```python
from build123d import *

# Parameters (mm, degrees)
SKETCH_2_R          = 4.5
CUT_EXTRUDE_1_DEPTH = 73.498275842


with BuildPart() as part:
    # 草图1 one side → 旋转4 (revolve)
    with BuildSketch(Plane(origin=(0, 0, 0), x_dir=(1, 0, 0), z_dir=(0, 1, 0)), mode=Mode.PRIVATE) as revolve_4_sk:
        with BuildLine():
            Line((0, 10), (-20.468871126, 10))
            ThreePointArc((-20.468871126, 10), (-23.116081379, 11.001287297), (-24.437982633, 13.503861062))
            Line((-24.437982633, 13.503861062), (-26, 26))
            Line((-26, 26), (-31, 26))
            Line((-31, 26), (-31, 10))
            Line((-31, 10), (-50, 10))
            Line((-50, 10), (-50, -2))
            Line((-50, -2), (-31, -2))
            Line((-31, -2), (-31, 0))
            Line((-31, 0), (0, 0))
            Line((0, 0), (0, 10))
        make_face()
    revolve(revolve_4_sk.sketch.rotate(Axis((0, 0, 0), (0, 0, -1)), 180), axis=Axis((0, 0, 0), (0, 0, -1)))

    # 草图2 → 切除-拉伸1 (cut, through all)
    with BuildSketch(Plane(origin=(0, 0, -10), x_dir=(-1, 0, 0), z_dir=(0, 0, -1))):
        with Locations((41, 0)):
            Circle(SKETCH_2_R)
        with Locations((0, -41)):
            Circle(SKETCH_2_R)
        with Locations((-41, 0)):
            Circle(SKETCH_2_R)
        with Locations((0, 41)):
            Circle(SKETCH_2_R)
    extrude(amount=-CUT_EXTRUDE_1_DEPTH, mode=Mode.SUBTRACT)


solid = part.part
```
Here's how the part is built. I have some questions about the finished solid (model axes, mm). A direction names the side the tool comes from. Coordinates: 2 decimals unless noted, no trailing zeros. Order: outer loops, then holes, each group sorted by start corner. A loop starts at its lowest first (then second) coordinate and runs counter-clockwise, first axis right, second up. Notation, with made-up numbers: (74, -31.75) - (88, -31.75) arc R22 ccw to (88, -4.75) - close; hole circle Ø11 at (18.5, -35). An arc over 180 degrees is marked (long way). One line per question, with ' | ' between items. Start each with the question number.
1. I'm going to push flat-ended pins straight in: pin 1 Ø1 at (x, z) = (16, -8.5) entering from +Y; pin 2 Ø1 at (x, z) = (24, -13) entering from +Y; pin 3 Ø6 at (x, y) = (17.5, 32.5) entering from -Z; pin 4 Ø7 at (x, y) = (41, 0) entering from -Z. Where does each tip first touch, or does it pass through?
2. If we section it at D-D (y = 43): Write out the boundary of the cut face in (x, z), and give its area (3 significant figures).
3. If we mould it in two halves opening along Z, with no side actions, what happens to faces 1 (the cylindrical face through (-4.036, -30.736, 0.986)), 2 (the flat face through (22, -23, 2)), 3 (the flat face through (16, 21, -26))? For each: released by +Z, released by -Z, zero draft, split by the parting line, or undercut.
4. Please list where these lines run through material, in increasing order: line 1 along Y through (x, z) = (0, 1.3); line 2 along Z through (x, y) = (-15.5, 12.5); line 3 along Z through (x, y) = (22.5, -39). Write a range as [from, to].
5. If we section it at A-A (x = 0): Write out the boundary of the cut face in (y, z), and give its area (3 significant figures).
6. Which directions (+Z, -Z, +X, -X, +Y, -Y) give clear straight access to the entire face, cutting with the end or side of a thin tool? Please do faces 4 (the flat face through (0, 0, 0)), 5 (the flat face through (0, 0, -10)), 6 (the cylindrical face through (36.708, 1.352, -4.084)).
7. If we section it at B-B (z = -2.5): Write out the boundary of the cut face in (x, y), and give its area (3 significant figures).
Model answer:
1) pin 1: stops at y = 47.54 | pin 2: stops at y = 20.22 | pin 3: stops at z = -10 | pin 4: passes through
2) outline: (-25.51, -10) - (-4.03, -10) - (-4.03, 2) - (-25.51, 2) - close; (4.03, -10) - (25.51, -10) - (25.51, 2) - (4.03, 2) - close | area: 516 mm²
3) face 1: zero draft | face 2: released by +Z | face 3: released by -Z
4) line 1: y = [-50, -45.5], [-36.5, -31], [31, 36.5], [45.5, 50] | line 2: z = [-10, 0] | line 3: z = [-10, 2]
5) outline: (-50, -10) - (-45.5, -10) - (-45.5, 2) - (-50, 2) - close; (-36.5, -10) - (-31, -10) - (-31, -26) - (-26, -26) - (-24.44, -13.5) arc R4 cw to (-20.47, -10) - (20.47, -10) arc R4 cw to (24.44, -13.5) - (26, -26) - (31, -26) - (31, -10) - (36.5, -10) - (36.5, 2) - (31, 2) - (31, 0) - (-31, 0) - (-31, 2) - (-36.5, 2) - close; (45.5, -10) - (50, -10) - (50, 2) - (45.5, 2) - close | area: 1,060 mm²
6) face 4: +Z | face 5: -Z | face 6: +Z, -Z
7) outline: circle Ø100 at (0, 0); hole circle Ø9 at (-41, 0); hole circle Ø9 at (0, -41); hole circle Ø9 at (0, 41); hole circle Ø9 at (41, 0) | area: 7,600 mm²
